Verification items for this drawing (mm, ordinates from the low corner). Coordinates: 2 decimals unless noted, no trailing zeros. Write each loop counter-clockwise with the first axis right and the second up, starting at its lowest first coordinate (ties: lowest second). Pieces come first, ordered by that corner, then holes. Notation, with made-up numbers: (22, 2.5) -> (79, 2.5) arc R11 cw to (79, 18.5) -> close; hole circle Ø7 at (60, -7). An arc over 180 degrees is marked (long way). One line per item, written item: value. Start each with the question number.
1) Sectioned sample at B-B on z = 10. Enter the section's corners in (x, y).
2) Sectioned sample at A-A on x = 10. Enter the section's corners in (y, z).
3) Scan lines: line 1 along Z through (x, y) = (10, 6.5); line 2 along X through (y, z) = (1.5, 58) (1 decimal); line 3 along Z through (x, y) = (93, 3) (1 decimal). Record each from-to range of solid material in increasing order. Write a range as [from, to].
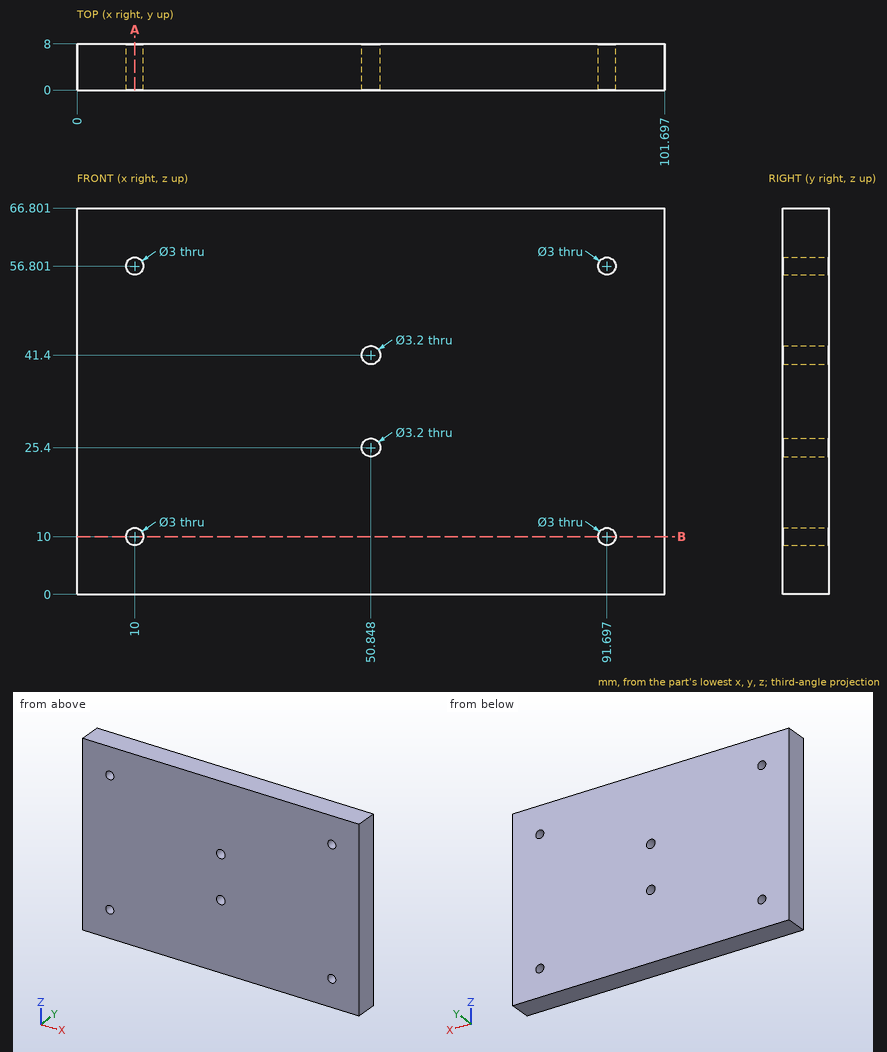
Answers:
1. outline: (0, 0) -> (8.5, 0) -> (8.5, 8) -> (0, 8) -> close; (11.5, 0) -> (90.2, 0) -> (90.2, 8) -> (11.5, 8) -> close; (93.2, 0) -> (101.7, 0) -> (101.7, 8) -> (93.2, 8) -> close
2. outline: (0, 0) -> (8, 0) -> (8, 8.5) -> (0, 8.5) -> close; (0, 11.5) -> (8, 11.5) -> (8, 55.3) -> (0, 55.3) -> close; (0, 58.3) -> (8, 58.3) -> (8, 66.8) -> (0, 66.8) -> close
3. line 1: z = [0, 8.5], [11.5, 55.3], [58.3, 66.8]
3. line 2: x = [0, 9.1], [10.9, 90.8], [92.6, 101.7]
3. line 3: z = [0, 9.3], [10.7, 56.1], [57.5, 66.8]
